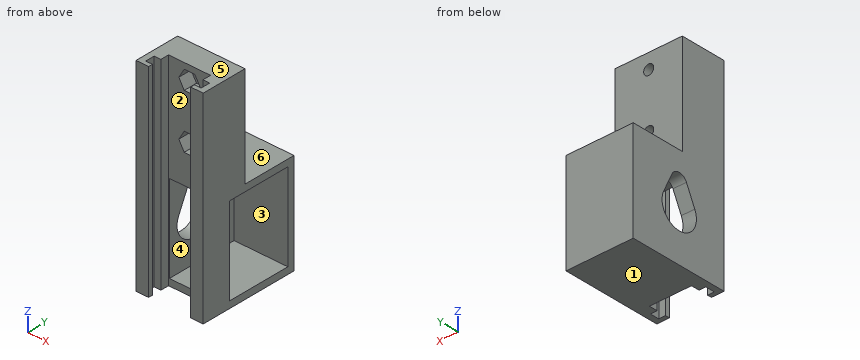
```python
from build123d import *

# Parameters (mm, degrees)
SKETCH1_W           = 20
SKETCH1_H           = 13.6
BOSS_EXTRUDE1_DEPTH = 65
SKETCH3_R           = 1.5
CUT_EXTRUDE2_DEPTH  = 68.298918099
SKETCH5_W           = 35
SKETCH5_H           = 5
CUT_EXTRUDE4_DEPTH  = 69.519668815
SKETCH6_W           = 12
SKETCH6_H           = 31
CUT_EXTRUDE5_DEPTH  = 5
SKETCH7_W           = 20
SKETCH7_H           = 35
BOSS_EXTRUDE2_DEPTH = 21
SKETCH8_W           = 31
SKETCH8_H           = 19
CUT_EXTRUDE6_DEPTH  = 16
CUT_EXTRUDE7_DEPTH  = 71.228177029
SKETCH11_W          = 5
SKETCH11_H          = 29.6
CUT_EXTRUDE8_DEPTH  = 72.246030408
BOSS_EXTRUDE3_REACH = 68.716
SKETCH12_W          = 2
SKETCH12_H          = 29.6
CUT_EXTRUDE9_DEPTH  = 65.576940359
CUT_EXTRUDE10_DEPTH = 4


with BuildPart() as part:
    # Sketch1 → Boss-Extrude1 (new body)
    with BuildSketch(Plane.XY):
        with Locations((0.917159763, -1.563313609)):
            Rectangle(SKETCH1_W, SKETCH1_H)
    extrude(amount=-BOSS_EXTRUDE1_DEPTH)

    # Sketch3 → Cut-Extrude2 (cut, through all)
    with BuildSketch(Plane(origin=(0, 5.236686391, 0), x_dir=(1, 0, 0), z_dir=(0, 1, 0))):
        with Locations(Location((0.917159763, 4.5, 0), (0, 0, 270))):
            Circle(SKETCH3_R)
        with Locations(Location((0.917159763, 20.589405581, 0), (0, 0, 270))):
            Circle(SKETCH3_R)
    extrude(amount=-CUT_EXTRUDE2_DEPTH, mode=Mode.SUBTRACT)

    # Sketch5 → Cut-Extrude4 (cut, through all)
    with BuildSketch(Plane(origin=(10.917159763, 0, 0), x_dir=(0, 0, -1), z_dir=(1, 0, 0))):
        with Locations((47.5, 2.736686391)):
            Rectangle(SKETCH5_W, SKETCH5_H)
    extrude(amount=-CUT_EXTRUDE4_DEPTH, mode=Mode.SUBTRACT)

    # Sketch6 → Cut-Extrude5 (cut)
    with BuildSketch(Plane(origin=(0, 0.236686391, 0), x_dir=(1, 0, 0), z_dir=(0, 1, 0))):
        with Locations((0.917159763, 47.5)):
            Rectangle(SKETCH6_W, SKETCH6_H)
    extrude(amount=-CUT_EXTRUDE5_DEPTH, mode=Mode.SUBTRACT)

    # Sketch7 → Boss-Extrude2 (add)
    with BuildSketch(Plane(origin=(0, 0.236686391, 0), x_dir=(1, 0, 0), z_dir=(0, 1, 0))):
        with Locations((0.917159763, 47.5)):
            Rectangle(SKETCH7_W, SKETCH7_H)
    extrude(amount=BOSS_EXTRUDE2_DEPTH)

    # Sketch8 → Cut-Extrude6 (cut)
    with BuildSketch(Plane(origin=(10.917159763, 0, 0), x_dir=(0, 0, -1), z_dir=(1, 0, 0))):
        with Locations((47.5, 9.736686391)):
            Rectangle(SKETCH8_W, SKETCH8_H)
    extrude(amount=-CUT_EXTRUDE6_DEPTH, mode=Mode.SUBTRACT)

    # Sketch9 → Cut-Extrude7 (cut, through all)
    with BuildSketch(Plane(origin=(-5.082840237, 0, 0), x_dir=(0, 0, -1), z_dir=(1, 0, 0))):
        with BuildLine():
            Line((37.385714286, 8.585806938), (43.1, 11.296330647))
            ThreePointArc((43.1, 11.296330647), (51.1, 6.236686391), (43.1, 1.177042134))
            Line((43.1, 1.177042134), (37.385714286, 3.887565843))
            ThreePointArc((37.385714286, 3.887565843), (35.9, 6.236686391), (37.385714286, 8.585806938))
        make_face()
    extrude(amount=-CUT_EXTRUDE7_DEPTH, mode=Mode.SUBTRACT)

    # Sketch11 → Cut-Extrude8 (cut, through all)
    with BuildSketch(Plane(origin=(10.917159763, 0, 0), x_dir=(0, 0, -1), z_dir=(1, 0, 0))):
        with Locations((62.5, 6.436686391)):
            Rectangle(SKETCH11_W, SKETCH11_H)
    extrude(amount=-CUT_EXTRUDE8_DEPTH, mode=Mode.SUBTRACT)

    # Boss-Extrude3: up to this face of the body (flat: up to its plane)
    boss_extrude3_end = Plane(part.part.faces().sort_by_distance((-9.082840237, 3.675844839, -34.656950913))[0])
    # Sketch12 → Boss-Extrude3 (add, up to the picked face)
    with BuildSketch(Plane(origin=(10.917159763, 0, 0), x_dir=(0, 0, -1), z_dir=(1, 0, 0)), mode=Mode.PRIVATE) as boss_extrude3_sk1:
        with Locations((59, 6.436686391)):
            Rectangle(SKETCH12_W, SKETCH12_H)
    boss_extrude3_tool1 = split(extrude(boss_extrude3_sk1.sketch, amount=-BOSS_EXTRUDE3_REACH, mode=Mode.PRIVATE), bisect_by=boss_extrude3_end, keep=Keep.BOTH, mode=Mode.PRIVATE)
    add(boss_extrude3_tool1.solids().sort_by(Axis((10.91716, 6.436686, -59), (-1, 0, 0)))[0])

    # Sketch2 → Cut-Extrude9 (cut, through all)
    with BuildSketch(Plane.XY):
        Polygon((-5.332840237, -8.363313609), (-5.332840237, -7.113313609), (-7.332840237, -7.113313609), (-7.332840237, -4.363313609), (-5.332840237, -4.363313609), (-5.332840237, -1.863313609), (7.167159763, -1.863313609), (7.167159763, -4.363313609), (9.167159763, -4.363313609), (9.167159763, -7.113313609), (7.167159763, -7.113313609), (7.167159763, -8.363313609), align=None)
    extrude(amount=-CUT_EXTRUDE9_DEPTH, mode=Mode.SUBTRACT)

    # Sketch13 → Cut-Extrude10 (cut)
    with BuildSketch(Plane.XZ.offset(1.863313609)):
        Polygon((2.507159763, -7.253960784), (4.097159763, -4.5), (2.507159763, -1.746039216), (-0.672840237, -1.746039216), (-2.262840237, -4.5), (-0.672840237, -7.253960784), align=None)
        Polygon((2.507159763, -23.343366365), (4.097159763, -20.589405581), (2.507159763, -17.835444797), (-0.672840237, -17.835444797), (-2.262840237, -20.589405581), (-0.672840237, -23.343366365), align=None)
    extrude(amount=-CUT_EXTRUDE10_DEPTH, mode=Mode.SUBTRACT)


solid = part.part
```
Read the model definition and answer for the solid it produces. Units are mm, in the model's axes. Face numbers are marked on the shaded views. A direction names the side the tool comes from. Give positions to 0.01 mm unless a question says otherwise; leave off trailing zeros. Loops run counter-clockwise (first coordinate to the right, second up) from the corner with the lowest first, then second, coordinate; pieces in that order, holes last.
Item 1: The mould has two halves that part along Z. Classify the marked faces 1, 2 and 3: released by +Z, released by -Z, zero draft, split by the parting line, or undercut.
Item 2: The part is cut by section D-D (z = -21.5). Write down the section's boundary in (x, y), and give its area (3 significant figures).
Item 3: The part is cut by section B-B (y = -5.75). Write down the section's boundary in (x, z).
Item 4: The part is cut by section A-A (z = -45.5). Write down the section's boundary in (x, y).
Item 5: For the marked faces 4, 5 and 6, determine the directions among +Z, -Z, +X, -X, +Y, -Y from which every point of the face is accessible in a straight line to the end or side of a thin tool.
Item 6: Each of these flat-tipped pins is pushed along its axis until it touches: pin 1 Ø10 at (x, y) = (-4, 14.5) entering from +Z; pin 2 Ø8 at (x, z) = (4, -45) entering from -Y; pin 3 Ø3 at (x, z) = (-6.5, -22) entering from +Y; pin 4 Ø2.5 at (x, z) = (0.92, -4.5) entering from +Y. Where does it stop, or does it pass through?
Item 7: Find the intervals of material crossed by line 1 along Z through (x, y) = (1, -0.25); line 2 along Z through (x, y) = (-4.5, 8.25); line 3 along Y through (x, z) = (-7.4, -45.5), in increasing order.
Item 8: The part is cut by section C-C (x = 6.25). Write down the section's boundary in (y, z).
Taken from the geometry:
1. face 1: released by -Z
1. face 2: zero draft
1. face 3: undercut
2. outline: (-9.08, -8.36) - (-5.33, -8.36) - (-5.33, -7.11) - (-7.33, -7.11) - (-7.33, -4.36) - (-5.33, -4.36) - (-5.33, -1.86) - (-1.74, -1.86) - (-1.74, 2.14) - (-0.27, 2.14) - (-0.27, 5.24) - (-9.08, 5.24) - close; (2.11, 2.14) - (3.57, 2.14) - (3.57, -1.86) - (7.17, -1.86) - (7.17, -4.36) - (9.17, -4.36) - (9.17, -7.11) - (7.17, -7.11) - (7.17, -8.36) - (10.92, -8.36) - (10.92, 5.24) - (2.11, 5.24) - close
2. area: 151 mm2
3. outline: (-9.08, -60) - (-7.33, -60) - (-7.33, 0) - (-9.08, 0) - close; (9.17, -60) - (10.92, -60) - (10.92, 0) - (9.17, 0) - close
4. outline: (-9.08, -8.36) - (-5.33, -8.36) - (-5.33, -7.11) - (-7.33, -7.11) - (-7.33, -4.36) - (-5.33, -4.36) - (-5.33, -1.86) - (-5.08, -1.86) - (-5.08, 0.64) - (-9.08, 0.64) - close; (-9.08, 11.84) - (-5.08, 11.84) - (-5.08, 19.24) - (10.92, 19.24) - (10.92, 21.24) - (-9.08, 21.24) - close; (6.92, -1.86) - (7.17, -1.86) - (7.17, -4.36) - (9.17, -4.36) - (9.17, -7.11) - (7.17, -7.11) - (7.17, -8.36) - (10.92, -8.36) - (10.92, 0.24) - (6.92, 0.24) - close
5. face 4: -Y
5. face 5: +Z, +X, -X, +Y, -Y
5. face 6: +Z, +X, -X, +Y
6. pin 1: stops at z = -30
6. pin 2: stops at y = -8.36
6. pin 3: stops at y = 5.24
6. pin 4: passes through
7. line 1: z = -60 to -58, -32 to -23.34, -17.84 to -7.25, -1.75 to 0
7. line 2: z = -60 to -58, -32 to -30
7. line 3: y = -8.36 to 0.64, 11.84 to 21.24
8. outline: (-1.86, -60) - (21.24, -60) - (21.24, -30) - (5.24, -30) - (5.24, 0) - (-1.86, 0) - (-1.86, -32) - (19.24, -32) - (19.24, -58) - (-1.86, -58) - close
